from build123d import *

# Parameters (mm, degrees)
F0_W     = 60
F0_H     = 34
F1_DEPTH = 7.9375
F3_D     = 4.318
F4_W     = 24.13
F4_H     = 12.7
F5_DEPTH = 7.9385


with BuildPart() as f1:
    # F0 (on Top) → F1 (new body)
    with BuildSketch(Plane.XY):
        Rectangle(F0_W, F0_H)
    extrude(amount=F1_DEPTH)

    # F3 (through all)
    with Locations(Plane.XY.offset(7.9375)):
        with Locations((0, 10), (0, -10)):
            Hole(F3_D / 2)

    # F4 (on face) → F5 (cut, through all)
    with BuildSketch(Plane.XY.offset(7.9375)):
        with Locations((-17.935, 10.65)):
            Rectangle(F4_W, F4_H)
        with Locations((17.935, 10.65)):
            Rectangle(F4_W, F4_H)
    extrude(amount=-F5_DEPTH, mode=Mode.SUBTRACT)


solid = f1.part
CAD build for the part. Positions are in the model's coordinates, mm. A direction names the side the tool comes from. Give positions to 0.01 mm unless a question says otherwise; leave off trailing zeros. Order: outer loops, then holes, each group sorted by start corner. A loop starts at its lowest first (then second) coordinate and runs counter-clockwise, first axis right, second up. Notation, with made-up numbers: (82.25, -38.5) - (127.25, -38.5) arc R19 cw to (127.25, -3.5) - close; hole circle Ø7 at (-23, -23). An arc over 180 degrees is marked (long way). Answer in a Markdown table with one row per item.
1. Saw through at D-D, the plane x = -8. Give the cut face in (y, z), plus the area to 3 significant figures.
Data:
| item | result |
|---|---|
| outline | (-17, 0) - (4.3, 0) - (4.3, 7.94) - (-17, 7.94) - close |
| area | 169 mm² |
2. Probe probe 1 along Y at (x, z) = (0, 6.75); probe 2 along Y at (x, z) = (27.5, 3); probe 3 along X at (y, z) = (-8.5, 4.25). List the from-to ranges inside material, lowest first. Write a range as [from, to].
Data:
| item | result |
|---|---|
| probe 1 | y = [-17, -12.16], [-7.84, 7.84], [12.16, 17] |
| probe 2 | y = [-17, 4.3] |
| probe 3 | x = [-30, -1.55], [1.55, 30] |
3. Pull direction X, two halves, no side cores. Call faces 4 (the flat face through (18, 4.3, 4)), 5 (the flat face through (30, -6, 4)), 6 (the cylindrical face through (0.28, 12.14, 3.91)): pulls with the +X half, pulls with the -X half, needs draft (parallel to the pull), parting line crosses it, or undercut.
Data:
| item | result |
|---|---|
| face 4 | needs draft |
| face 5 | pulls with the +X half |
| face 6 | undercut |
4. Tool access for faces 1 (the flat face through (0, -17, 4)), 2 (the flat face through (5.87, 11, 4)), 3 (the flat face through (-5.87, 11, 4)): list every direction of +Z, -Z, +X, -X, +Y, -Y with a clear straight run to the whole face (end or side of a thin tool).
Data:
| item | result |
|---|---|
| face 1 | +Z, -Z, +X, -X, -Y |
| face 2 | +Z, -Z, +X, +Y |
| face 3 | +Z, -Z, -X, +Y |
5. Flat gauge pins, fed straight in: pin 1 (5 mm diameter, centred on x = 0, y = -10, fed in from -Z); pin 2 (4 mm diameter, centred on x = -21, z = 3.5, fed in from +Y). Where does each tip first touch, or does it go through?
Data:
| item | result |
|---|---|
| pin 1 | stops at z = 0 |
| pin 2 | stops at y = 4.3 |
6. Saw through at B-B, the plane z = 2.25. Give the cut face in (x, y), plus the area to 3 significant figures.
Data:
| item | result |
|---|---|
| outline | (-30, -17) - (30, -17) - (30, 4.3) - (5.87, 4.3) - (5.87, 17) - (-5.87, 17) - (-5.87, 4.3) - (-30, 4.3) - close; hole circle Ø4.32 at (0, -10); hole circle Ø4.32 at (0, 10) |
| area | 1,400 mm² |
7. Saw through at C-C, the plane y = 10. Give the cut face in (x, z), plus the area to 3 significant figures.
Data:
| item | result |
|---|---|
| outline | (-5.87, 0) - (-2.16, 0) - (-2.16, 7.94) - (-5.87, 7.94) - close; (2.16, 0) - (5.87, 0) - (5.87, 7.94) - (2.16, 7.94) - close |
| area | 58.9 mm² |
8. Saw through at A-A, the plane y = -10. Give the cut face in (x, z).
Data:
| item | result |
|---|---|
| outline | (-30, 0) - (-2.16, 0) - (-2.16, 7.94) - (-30, 7.94) - close; (2.16, 0) - (30, 0) - (30, 7.94) - (2.16, 7.94) - close |
